Can you work these out from the drawing? Everything is in mm from the part's minimum corner. A direction names the side the tool comes from. Give positions to 0.01 mm unless a question says otherwise; leave off trailing zeros. Loops run counter-clockwise (first coordinate to the right, second up) from the corner with the lowest first, then second, coordinate; pieces in that order, holes last. Notation, with made-up numbers: (19.25, 50) - (36.25, 50) arc R12 ccw to (36.25, 67) - close; hole circle Ø10 at (63, 52). An arc over 180 degrees is marked (long way). Answer in a Markdown table with one row per item.
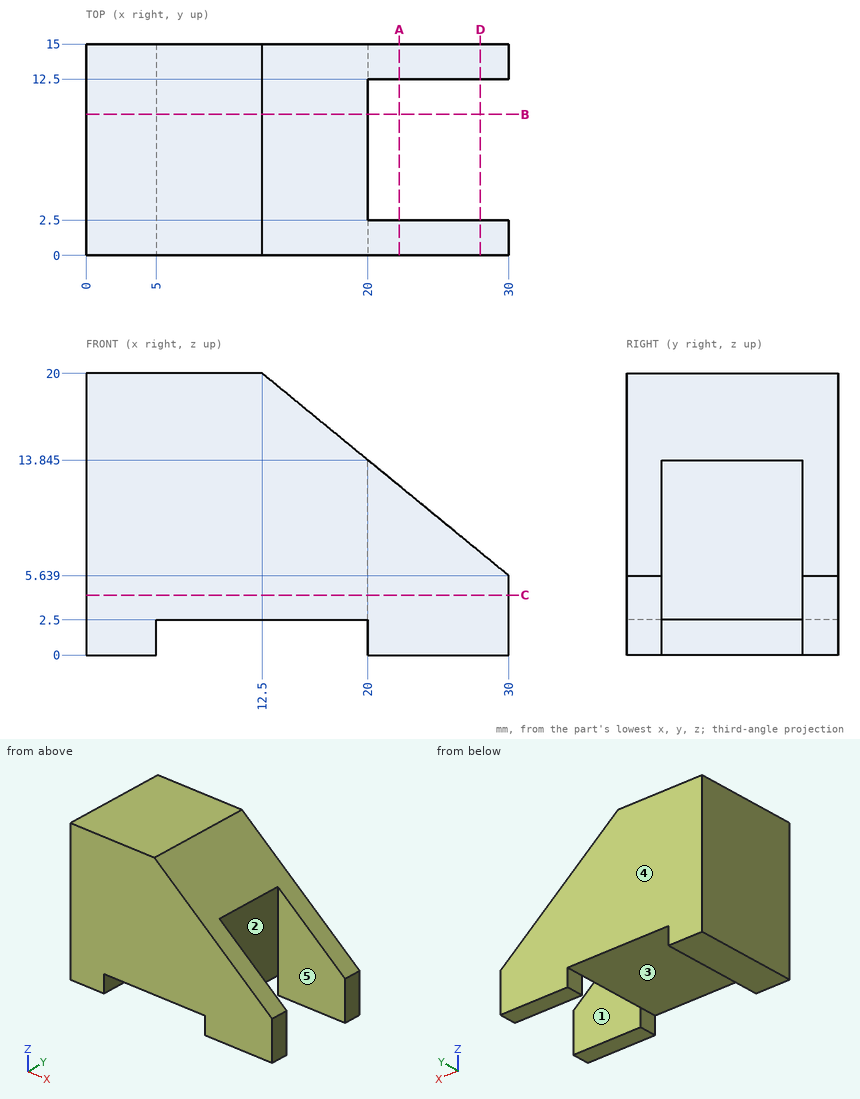
Q1. If I drill on line 1 (X direction, y = 13.5, z = 1.75); line 2 (Y direction, x = 22.5, z = 8); line 3 (X direction, y = 8, z = 13), over which ranges is the centre line in solid material (lowest first)? Write a range as [from, to].
Checked values:
| item | result |
|---|---|
| line 1 | x = [0, 5], [20, 30] |
| line 2 | y = [0, 2.5], [12.5, 15] |
| line 3 | x = [0, 20] |
Q2. On a 3-axis mill with a long thin cutter (end or side, diameter ignored), from which of +Z, -Z, +X, -X, +Y, -Y can I reach the whole of each face in a straight line? I mean the marked faces 4 and 5. Say none if no direction works.
Checked values:
| item | result |
|---|---|
| face 4 | +Z, -Z, +X, -X, +Y |
| face 5 | +Z, -Z, +X |
Q3. If we mould it in two halves opening along X, with no side actions, what happens to the marked faces 1, 2 and 3? For each: released by +X, released by -X, zero draft, split by the parting line, or undercut.
Checked values:
| item | result |
|---|---|
| face 1 | zero draft |
| face 2 | released by +X |
| face 3 | undercut |
Q4. Imagine slicing it at A-A, the plane x = 22.25. Write out the boundary of the cut face in (y, z), and give its area (3 significant figures).
Checked values:
| item | result |
|---|---|
| outline | (0, 0) - (2.5, 0) - (2.5, 12) - (0, 12) - close; (12.5, 0) - (15, 0) - (15, 12) - (12.5, 12) - close |
| area | 60.0 mm² |
Q5. Imagine slicing it at D-D, the plane x = 28. Write out the boundary of the cut face in (y, z), and give its area (3 significant figures).
Checked values:
| item | result |
|---|---|
| outline | (0, 0) - (2.5, 0) - (2.5, 7.28) - (0, 7.28) - close; (12.5, 0) - (15, 0) - (15, 7.28) - (12.5, 7.28) - close |
| area | 36.4 mm² |
Q6. Imagine slicing it at B-B, the plane y = 10. Write out the boundary of the cut face in (x, z) (1 decimal).
Checked values:
| item | result |
|---|---|
| outline | (0, 0) - (5, 0) - (5, 2.5) - (20, 2.5) - (20, 13.8) - (12.5, 20) - (0, 20) - close |
Q7. Imagine slicing it at C-C, the plane z = 4.25. Write out the boundary of the cut face in (x, y).
Checked values:
| item | result |
|---|---|
| outline | (0, 0) - (30, 0) - (30, 2.5) - (20, 2.5) - (20, 12.5) - (30, 12.5) - (30, 15) - (0, 15) - close |
Q8. For pin 1 (7.5 mm diameter, centred on x = 9, y = 4, fed in from -Z); pin 2 (4 mm diameter, centred on y = 9.5, z = 17, fed in from +X); pin 3 (1.2 mm diameter, centred on y = 8, z = 1, fed in from +X), each with a flat end and sliding along its axis, tell me the tip position at first contact or that it passes through.
Checked values:
| item | result |
|---|---|
| pin 1 | stops at z = 2.5 |
| pin 2 | stops at x = 18.59 |
| pin 3 | stops at x = 5 |
